from build123d import *


with BuildPart() as part:
    # Эскиз1 → Повернуть1 (revolve)
    with BuildSketch(Plane.XY):
        with BuildLine():
            Line((6.428300829, 12.5), (-8.571699171, 12.5))
            Line((-8.571699171, 12.5), (-8.571699171, 26))
            Line((-8.571699171, 26), (-13.071699171, 26))
            Line((-13.071699171, 26), (-13.071699171, 30))
            Line((-13.071699171, 30), (-8.071699171, 30))
            Line((-8.071699171, 30), (-8.071699171, 65.5))
            ThreePointArc((-8.071699171, 65.5), (-7.485912733, 66.914213562), (-6.071699171, 67.5))
            Line((-6.071699171, 67.5), (6.071699171, 67.5))
            ThreePointArc((6.071699171, 67.5), (7.432388365, 66.965784745), (8.066176633, 65.648524917))
            Line((8.066176633, 65.648524917), (11.428300829, 20.5))
            Line((11.428300829, 20.5), (6.428300829, 20.5))
            Line((6.428300829, 20.5), (6.428300829, 12.5))
        make_face()
    revolve(axis=Axis((-643.332684128, 0, 0), (1, 0, 0)))


solid = part.part
Build history of the part. All positions in model axes, mm. A direction names the side the tool comes from. Round coordinates to 2 decimals unless told otherwise and drop trailing zeros. Loops run counter-clockwise (first coordinate to the right, second up) from the corner with the lowest first, then second, coordinate; pieces in that order, holes last. Notation, with made-up numbers: (83, 49) -> (137, 49) arc R13 ccw to (137, 70) -> close; hole circle Ø2 at (-2, 8). An arc over 180 degrees is marked (long way). One line per item, written item: value. Start each with the question number.
Q1. Cut at C-C on x = 4.25. List the corners of the cut face in (y, z).
Q2. Drop flat-ended pins along their axis: pin 1 Ø8 at (x, y) = (-8, 20) entering from +Z; pin 2 Ø12 at (x, y) = (-8.5, -41.5) entering from +Z; pin 3 Ø2 at (x, y) = (3, -20) entering from +Z. Give the stop position or say it passes through.
Q3. Two-plate mould, pull along Y, no slides. Class faces 3 (the face through (-10.54, -29.97, 1.32)), 4 (the face through (-8.072, -14, -28)), 5 (the face through (-8.572, -11.2, 6.1)), 6 (the face through (-10.853, -20.633, -15.821)): released by +Y, released by -Y, zero draft, split by the parting line, or undercut.
Q4. 3-axis set-ups, long thin cutter, end or side, ignore diameter. For faces 1 (the face through (8.893, -4.444, -20.013)), 2 (the face through (-13.072, 9, 25)): which of +Z, -Z, +X, -X, +Y, -Y reach the whole face in a straight line?
Q5. Cut at A-A on z = 0. List the corners of the cut face in (x, y).
Q6. Probe line 1 along Z through (x, y) = (0.5, 0); line 2 along Z through (x, y) = (-12.15, 0); line 3 along X through (y, z) = (-18, -2.5). List the from-to ranges inside material, lowest first.
Computed:
1. outline: circle Ø135 at (0, 0); hole circle Ø25 at (0, 0)
2. pin 1: z = 65.47
2. pin 2: z = 57.14
2. pin 3: z = 64.77
3. face 3: split by the parting line
3. face 4: zero draft
3. face 5: undercut
3. face 6: undercut
4. face 1: +X
4. face 2: +Z, -Z, -X, +Y, -Y
5. outline: (-13.07, -30) -> (-8.07, -30) -> (-8.07, -65.5) arc R2 ccw to (-6.07, -67.5) -> (6.07, -67.5) arc R2 ccw to (8.07, -65.65) -> (11.43, -20.5) -> (6.43, -20.5) -> (6.43, -12.5) -> (-8.57, -12.5) -> (-8.57, -26) -> (-13.07, -26) -> close; (-13.07, 26) -> (-8.57, 26) -> (-8.57, 12.5) -> (6.43, 12.5) -> (6.43, 20.5) -> (11.43, 20.5) -> (8.07, 65.65) arc R2 ccw to (6.07, 67.5) -> (-6.07, 67.5) arc R2 ccw to (-8.07, 65.5) -> (-8.07, 30) -> (-13.07, 30) -> close
6. line 1: -67.5 to -12.5, 12.5 to 67.5
6. line 2: -30 to -26, 26 to 30
6. line 3: -8.57 to 6.43
